```python
from build123d import *

# Parameters (mm, degrees)
ESQUISSE1_W     = 40
ESQUISSE1_H     = 30
ESQUISSE1_R     = 2
BASE_DEPTH      = 5
EXT_R           = 5
ESQUISSE2_R     = 4
ACCES_VIS_DEPTH = 2.5


with BuildPart() as part:
    # Esquisse1 → BASE (new body)
    with BuildSketch(Plane(origin=(0, 0, 0), x_dir=(1, 0, 0), z_dir=(0, 1, 0))):
        Rectangle(ESQUISSE1_W, ESQUISSE1_H)
        with Locations(Location((0, 0, 0), (0, 0, 270))):
            Circle(ESQUISSE1_R, mode=Mode.SUBTRACT)
    extrude(amount=BASE_DEPTH)

    # EXT
    ext_edges = [part.edges().sort_by_distance(p)[0] for p in [
        (-20, 0, 0),
        (0, 0, -15),
        (20, 0, 0),
        (0, 0, 15),
    ]]
    fillet(ext_edges, radius=EXT_R - 0.0001)  # a hair under: the kernel refuses the full size

    # Esquisse2 → ACCES VIS (cut)
    with BuildSketch(Plane(origin=(0, 0, 0), x_dir=(-1, 0, 0), z_dir=(0, -1, 0))):
        with Locations(Location((0, 0, 0), (0, 0, 90))):
            Circle(ESQUISSE2_R)
    extrude(amount=-ACCES_VIS_DEPTH, mode=Mode.SUBTRACT)


solid = part.part
```
Check sheet for the modelled part. Datum: model origin and axes. Units: mm. A direction names the side the tool comes from. Round coordinates to 2 decimals unless told otherwise and drop trailing zeros. Order: outer loops, then holes, each group sorted by start corner. A loop starts at its lowest first (then second) coordinate and runs counter-clockwise, first axis right, second up.
1) Scan lines: line 1 (Y direction, x = 1, z = 2.5); line 2 (X direction, y = 1.25, z = -0.75); line 3 (Z direction, x = -8, y = 4.7). Record each from-to range of solid material in increasing order.
2) Go/stop test with flat-tipped pins: pin 1 Ø1 at (x, y) = (-2, 0.5) entering from -Z; pin 2 Ø2 at (y, z) = (0.5, -5.5) entering from -X; pin 3 Ø2 at (x, y) = (6, 3.5) entering from -Z. Record where each tip stops, or that it passes through.
3) Section check C-C (y = 1.1). Record the boundary of the cut face in (x, z), and give its area (3 significant figures).
4) Tool access check on faces 1 (the flat face through (-1, 2.5, 2)), 2 (the flat face through (-4, 0, -2)). Record the directions out of +Z, -Z, +X, -X, +Y, -Y that give a thin tool (end or side, any length) a straight path to the whole face; none if there is none.
5) Mould release check, pull along X, two halves, no side actions. Record for faces 3 (the flat face through (0, 5, -4)), 4 (the cylindrical face through (-19, 2, 0)), 5 (the cylindrical face through (-2, 4, 0)), 6 (the cylindrical face through (19, 2, 0)): +X half, -X half, draft (parallel to the pull), parting line (faces both ways), or undercut.
Result:
1. line 1: y = 2.5 to 5
1. line 2: x = -18.31 to -3.93, 3.93 to 18.31
1. line 3: z = -14.99 to 14.99
2. pin 1: stops at z = -13
2. pin 2: stops at x = -18.57
2. pin 3: stops at z = -14.97
3. outline: (-18.13, -13.13) - (18.13, -13.13) - (18.13, 13.13) - (-18.13, 13.13) - close; hole circle Ø8 at (0, 0)
3. area: 902 mm2
4. face 1: -Y
4. face 2: +Z, -Z, +X, -X, -Y
5. face 3: draft
5. face 4: -X half
5. face 5: undercut
5. face 6: +X half
